Model file for the job. Use its own axes, mm. A direction names the side the tool comes from. Coordinates: 2 decimals unless noted, no trailing zeros. Write each loop counter-clockwise with the first axis right and the second up, starting at its lowest first coordinate (ties: lowest second). Pieces come first, ordered by that corner, then holes. Notation, with made-up numbers: (72, 10.5) -> (117, 10.5) arc R19 ccw to (117, 31.5) -> close; hole circle Ø2 at (-32, 84). An arc over 180 degrees is marked (long way). Write item = value, one per line. Start each with the question number.
from build123d import *

# Parameters (mm, degrees)
F0_R     = 40.64
F0_R_2   = 37.765528
F1_DEPTH = 127
F3_DEPTH = 40.641
F4_DEPTH = 76.2
F5_DEPTH = 50.8
F6_DEPTH = 50.8
F8_DEPTH = 50.8
F9_DEPTH = 50.8


with BuildPart() as f1:
    # F0 (on Top) → F1 (new body)
    with BuildSketch(Plane.XY):
        Circle(F0_R)
        Circle(F0_R_2, mode=Mode.SUBTRACT)
    extrude(amount=F1_DEPTH)

    # F2 (on Front) → F3 (cut, through all)
    with BuildSketch(Plane.XZ):
        with BuildLine():
            ThreePointArc((20.893278, 93.254258), (17.083276, 97.064259), (13.273275, 93.254258))
            Line((13.273275, 93.254258), (13.273275, 64.494903))
            ThreePointArc((13.273275, 64.494903), (17.083276, 60.684902), (20.893278, 64.494903))
            Line((20.893278, 64.494903), (20.893278, 93.254258))
        make_face()
    extrude(amount=-F3_DEPTH, mode=Mode.SUBTRACT)

    # F2 (on Front) → F4 (cut)
    with BuildSketch(Plane.XZ):
        with BuildLine():
            ThreePointArc((-10.815753, 97.929251), (-14.625754, 101.739253), (-18.435756, 97.929251))
            Line((-18.435756, 97.929251), (-18.435756, 69.169897))
            ThreePointArc((-18.435756, 69.169897), (-14.625754, 65.359895), (-10.815753, 69.169897))
            Line((-10.815753, 69.169897), (-10.815753, 97.929251))
        make_face()
    extrude(amount=-F4_DEPTH, mode=Mode.SUBTRACT)

    # F2 (on Front) → F5 (cut)
    with BuildSketch(Plane.XZ):
        with BuildLine():
            ThreePointArc((-18.927373, 16.02255), (-17.811449, 13.328472), (-15.117371, 12.212548))
            ThreePointArc((-15.117371, 12.212548), (-12.423293, 13.328472), (-11.307369, 16.02255))
            Line((-11.307369, 16.02255), (-11.307369, 44.781905))
            ThreePointArc((-11.307369, 44.781905), (-15.117371, 48.591906), (-18.927373, 44.781905))
            Line((-18.927373, 44.781905), (-18.927373, 16.02255))
        make_face()
    extrude(amount=F5_DEPTH, mode=Mode.SUBTRACT)

    # F2 (on Front) → F6 (cut)
    with BuildSketch(Plane.XZ):
        with BuildLine():
            ThreePointArc((24.211667, 44.781905), (20.401666, 48.591906), (16.591664, 44.781905))
            Line((16.591664, 44.781905), (16.591664, 16.02255))
            ThreePointArc((16.591664, 16.02255), (17.707588, 13.328472), (20.401666, 12.212548))
            ThreePointArc((20.401666, 12.212548), (23.095744, 13.328472), (24.211667, 16.02255))
            Line((24.211667, 16.02255), (24.211667, 44.781905))
        make_face()
    extrude(amount=F6_DEPTH, mode=Mode.SUBTRACT)

    # F7 (on Right) → F8 (cut)
    with BuildSketch(Plane.YZ):
        with BuildLine():
            ThreePointArc((-5.653547, 115.610962), (-9.463548, 119.420963), (-13.27355, 115.610962))
            Line((-13.27355, 115.610962), (-13.27355, 86.851607))
            ThreePointArc((-13.27355, 86.851607), (-9.463548, 83.041606), (-5.653547, 86.851607))
            Line((-5.653547, 86.851607), (-5.653547, 115.610962))
        make_face()
    extrude(amount=-F8_DEPTH, mode=Mode.SUBTRACT)

    # F7 (on Right) → F9 (cut)
    with BuildSketch(Plane.YZ):
        with BuildLine():
            ThreePointArc((-5.653547, 115.610962), (-9.463548, 119.420963), (-13.27355, 115.610962))
            Line((-13.27355, 115.610962), (-13.27355, 86.851607))
            ThreePointArc((-13.27355, 86.851607), (-9.463548, 83.041606), (-5.653547, 86.851607))
            Line((-5.653547, 86.851607), (-5.653547, 115.610962))
        make_face()
        with BuildLine():
            ThreePointArc((-28.021937, 93.734198), (-31.831939, 97.5442), (-35.64194, 93.734198))
            Line((-35.64194, 93.734198), (-35.64194, 64.974844))
            ThreePointArc((-35.64194, 64.974844), (-31.831939, 61.164842), (-28.021937, 64.974844))
            Line((-28.021937, 64.974844), (-28.021937, 93.734198))
        make_face()
        with BuildLine():
            ThreePointArc((23.351614, 116.102581), (19.541613, 119.912582), (15.731611, 116.102581))
            Line((15.731611, 116.102581), (15.731611, 87.343226))
            ThreePointArc((15.731611, 87.343226), (19.541613, 83.533225), (23.351614, 87.343226))
            Line((23.351614, 87.343226), (23.351614, 116.102581))
        make_face()
    extrude(amount=-F9_DEPTH, mode=Mode.SUBTRACT)


solid = f1.part
(1) 3-axis set-ups, long thin cutter, end or side, ignore diameter. For faces 5 (the face through (13.273, 37, 79)), 6 (the face through (-33.522, 19.458, 83.534)), 7 (the face through (-11.307, -38, 30)), 8 (the face through (-18.927, -34, 31)), 9 (the face through (-14.54, 36.02, 101.74)): which of +Z, -Z, +X, -X, +Y, -Y reach the whole face in a straight line?
(2) Saw through at B-B (z = 103.5). Give the cut face in (x, y).
(3) Mould opens along Y. For faces 1 (the face through (-37.77, -9.38, 119.42)), 2 (the face through (24.212, -31, 30)), 3 (the face through (-36, 15.732, 102)), 4 (the face through (-27, -28.022, 79)) say: released by +Y, released by -Y, zero draft, split by the parting line, or undercut.
(4) Drop flat-ended pins along their axis: pin 1 Ø4 at (y, z) = (-31, 24.5) entering from -X; pin 2 Ø3.5 at (y, z) = (36.5, 78) entering from +X; pin 3 Ø2.5 at (y, z) = (37.5, 89) entering from -X; pin 4 Ø4 at (x, y) = (-27, -22) entering from +Z. Give the stop position or say it passes through.
(5) Drill centre lines: line 1 along Y through (x, z) = (0, 36.5); line 2 along X through (y, z) = (-33.5, 58.5); line 3 along Y through (x, z) = (-27.5, 35). Where is each one in solid material? Low to high.
(6) Saw through at A-A (x = 0). Give the cut face in (y, z), then the cut area to 3 significant figures.
Returned:
q1.face_5 = +X, +Y
q1.face_6 = -X
q1.face_7 = -X, -Y
q1.face_8 = -Y
q1.face_9 = +Y
q2.outline = (-40.24, -5.65) -> (-37.34, -5.65) arc R37.77 cw to (-34.33, 15.73) -> (-37.47, 15.73) arc R40.64 ccw to start; (-38.41, -13.27) arc R40.64 ccw (long way) to (-33.26, 23.35) -> (-29.68, 23.35) arc R37.77 cw (long way) to (-35.36, -13.27) -> close
q3.face_1 = undercut
q3.face_2 = zero draft
q3.face_3 = released by +Y
q3.face_4 = released by -Y
q4.pin_1 = -28.47
q4.pin_2 = 21.07
q4.pin_3 = -10.82
q4.pin_4 = through
q5.line_1 = -40.64 to -37.77, 37.77 to 40.64
q5.line_2 = -23.01 to -17.44, 17.44 to 23.01
q5.line_3 = -29.92 to -25.88, 25.88 to 29.92
q6.outline = (-40.64, 0) -> (-37.77, 0) -> (-37.77, 127) -> (-40.64, 127) -> close; (37.77, 0) -> (40.64, 0) -> (40.64, 127) -> (37.77, 127) -> close
q6.area = 730 mm2
